from build123d import *

# Parameters (mm, degrees)
F1_DEPTH = 12.7
F2_SIZE  = 0.762
F4_R     = 3.175
F5_DEPTH = 25.401


with BuildPart() as f1:
    # F0 (on Right) → F1 (new body)
    with BuildSketch(Plane.YZ):
        with BuildLine():
            ThreePointArc((-45.125007, 46.633742), (-46.023033, 46.261768), (-46.395007, 45.363742))
            Line((-46.395007, 45.363742), (-46.395007, 30.123742))
            ThreePointArc((-46.395007, 30.123742), (-46.023033, 29.225717), (-45.125007, 28.853742))
            Line((-45.125007, 28.853742), (-29.885007, 28.853742))
            ThreePointArc((-29.885007, 28.853742), (-28.986982, 29.225717), (-28.615007, 30.123742))
            Line((-28.615007, 30.123742), (-28.615007, 45.363742))
            ThreePointArc((-28.615007, 45.363742), (-28.986982, 46.261768), (-29.885007, 46.633742))
            Line((-29.885007, 46.633742), (-45.125007, 46.633742))
        make_face()
    extrude(amount=F1_DEPTH)

    # F2
    f2_edges = [f1.edges().sort_by_distance(p)[0] for p in [
        (0, -37.505007, 46.633742),
        (0, -46.395007, 37.743742),
    ]]
    chamfer(f2_edges, length=F2_SIZE)

    # F3: F1 across plane


with BuildPart() as f1_1:
    add(f1.part)
    add(f1.part.mirror(Plane.YZ))

    # F4 (on face) → F5 (cut, through all)
    with BuildSketch(Plane.YZ.offset(12.7)):
        with Locations((-37.505007, 38.162194)):
            Circle(F4_R)
    extrude(amount=-F5_DEPTH, mode=Mode.SUBTRACT)


solid = f1_1.part
Could you check a few things on this model? Use its own coordinates, in mm. A direction names the side the tool comes from. Round coordinates to 2 decimals unless told otherwise and drop trailing zeros. Order: outer loops, then holes, each group sorted by start corner. A loop starts at its lowest first (then second) coordinate and runs counter-clockwise, first axis right, second up. Notation, with made-up numbers: M -24.5,73.5 L -7.5,73.5 A34 cw -7.5,111.5 Z; hole C -39.5,64.5 d1. An arc over 180 degrees is marked long. One line per item, written item: value.
(1) I need wall thicknesses on line 1 along X through (y, z) = (-36.25, 46.25); line 2 along Y through (x, z) = (-9, 38) (3 decimals); line 3 along Y through (x, z) = (-4.5, 39.25) (3 decimals). Which ranges of each line are inside material? Lowest first, please. Write a range as from..to.
Ans:
line 1: x = -12.7..-0.38, 0.38..12.7
line 2: y = -46.395..-40.676, -34.334..-28.615
line 3: y = -46.395..-40.488, -34.522..-28.615
(2) If we mould it in two halves opening along Y, with no side actions, what happens to faces 4 (the flat face through (7, -28.615, 38)), 5 (the flat face through (-7, -37, 46.634)), 6 (the cylindrical face through (6.647, -46.013, 46.272)), 7 (the cylindrical face through (0.178, -36.04, 35.345))? For each: released by +Y, released by -Y, zero draft, split by the parting line, or undercut.
Ans:
face 4: released by +Y
face 5: zero draft
face 6: released by -Y
face 7: undercut
(3) Imagine slicing it at B-B (y = -38.5). Write out the boundary of the cut face in (x, z), and give its area (3 significant figures).
Ans:
outline: M -12.7,28.85 L -0.76,28.85 L 0,29.62 L 0.76,28.85 L 12.7,28.85 L 12.7,35.15 L -12.7,35.15 Z; M -12.7,41.18 L 12.7,41.18 L 12.7,46.63 L 0.76,46.63 L 0,45.87 L -0.76,46.63 L -12.7,46.63 Z
area: 297 mm^2
(4) Which directions (+Z, -Z, +X, -X, +Y, -Y) give clear straight access to the entire face, cutting with the end or side of a thin tool? Please do faces 1 (the conical face through (-0.291, -45.684, 45.935)), 2 (the conical face through (0.29, -29.33, 29.55)), 3 (the cylindrical face through (6.647, -28.997, 29.216)).
Ans:
face 1: +Z, -Y
face 2: -Z, +Y
face 3: -Z, +X, -X, +Y
(5) Imagine slicing it at A-A (z = 40). Write out the boundary of the cut face in (x, y) (3 decimals), and give its area (3 significant figures).
Ans:
outline: M -12.7,-46.395 L -0.762,-46.395 L 0,-45.633 L 0.762,-46.395 L 12.7,-46.395 L 12.7,-40.094 L -12.7,-40.094 Z; M -12.7,-34.916 L 12.7,-34.916 L 12.7,-28.615 L 0.762,-28.615 L 0,-29.377 L -0.762,-28.615 L -12.7,-28.615 Z
area: 319 mm^2
(6) Imagine slicing it at C-C (x = -7). Write out the boundary of the cut face in (y, z) (3 decimals), and give its area (3 significant figures).
Ans:
outline: M -46.395,30.124 A1.27 ccw -45.125,28.854 L -29.885,28.854 A1.27 ccw -28.615,30.124 L -28.615,45.364 A1.27 ccw -29.885,46.634 L -45.125,46.634 A1.27 ccw -46.395,45.364 Z; hole C -37.505,38.162 d6.35
area: 283 mm^2
